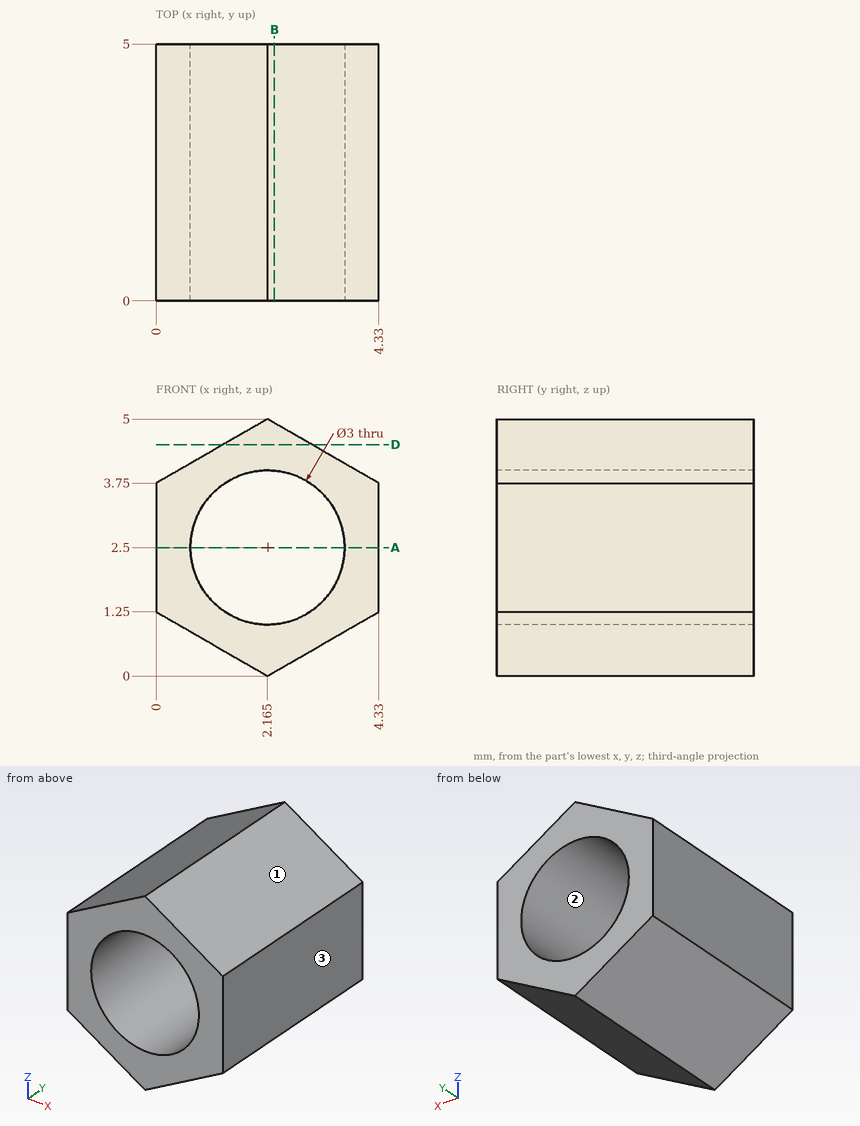
For this review, use the dimensioned drawing (mm, ordinates from the lowest corner) and the shaded views. Round coordinates to 2 decimals unless told otherwise and drop trailing zeros. Write each loop counter-clockwise with the first axis right and the second up, starting at its lowest first coordinate (ties: lowest second). Pieces come first, ordered by that corner, then holes. Notation, with made-up numbers: (-1.75, 76.25) - (10.25, 76.25) arc R13 ccw to (10.25, 97.25) - close; hole circle Ø7 at (8.5, -2). An arc over 180 degrees is marked (long way). Use a Markdown table: item, result.
Q1. We need section D-D (z = 4.5). Give the boundary of the cut face in (x, y).
Derived:
| item | result |
|---|---|
| outline | (1.3, 0) - (3.03, 0) - (3.03, 5) - (1.3, 5) - close |
Q2. We need section B-B (x = 2.3). Give the boundary of the cut face in (y, z).
Derived:
| item | result |
|---|---|
| outline | (0, 0.08) - (5, 0.08) - (5, 1.01) - (0, 1.01) - close; (0, 3.99) - (5, 3.99) - (5, 4.92) - (0, 4.92) - close |
Q3. Wall thickness on line 1 along X through (y, z) = (1.7, 3.4) (1 decimal); line 2 along X through (y, z) = (3.05, 1.8); line 3 along Z through (x, y) = (3.1, 0.55): over which ranges is each line inside the solid? List them lowest first.
Derived:
| item | result |
|---|---|
| line 1 | x = 0 to 1, 3.4 to 4.3 |
| line 2 | x = 0 to 0.84, 3.49 to 4.33 |
| line 3 | z = 0.54 to 1.33, 3.67 to 4.46 |
Q4. Clearance check with flat-ended pins moving along their axes: pin 1 (2 mm diameter, centred on y = 3.5, z = 3, fed in from -X); pin 2 (1 mm diameter, centred on x = 1.5, y = 2.5, fed in from -Z) (1 decimal). State where each tip first meets the part, or that it passes through.
Derived:
| item | result |
|---|---|
| pin 1 | stops at x = 0 |
| pin 2 | stops at z = 0.1 |
Q5. The part is to be moulded in two halves that separate along Z. For the marked faces 1, 2 and 3, say which applies: pulls with the +Z half, pulls with the -Z half, needs draft (parallel to the pull), parting line crosses it, or undercut.
Derived:
| item | result |
|---|---|
| face 1 | pulls with the +Z half |
| face 2 | undercut |
| face 3 | needs draft |
Q6. We need section A-A (z = 2.5). Give the boundary of the cut face in (x, y) (1 decimal).
Derived:
| item | result |
|---|---|
| outline | (0, 0) - (0.7, 0) - (0.7, 5) - (0, 5) - close; (3.7, 0) - (4.3, 0) - (4.3, 5) - (3.7, 5) - close |
